Read the model definition and answer for the solid it produces. Units are mm, in the model's axes. A direction names the side the tool comes from. Give positions to 0.01 mm unless a question says otherwise; leave off trailing zeros. Order: outer loops, then holes, each group sorted by start corner. A loop starts at its lowest first (then second) coordinate and runs counter-clockwise, first axis right, second up.
Item 1: Find the intervals of material crossed by line 1 along Z through (x, y) = (-67, 215); line 2 along Z through (x, y) = (-125, 37); line 3 along Y through (x, z) = (-145.5, -16.5), in increasing order.
Item 2: Given pin 1 Ø2 at (x, y) = (-131, 12) entering from -Z; pin 2 Ø15.5 at (x, z) = (-147, -16) entering from +Y; pin 3 Ø1 at (y, z) = (132.5, -10.5) entering from +X; pin 4 Ø1.5 at (x, y) = (-107, 18) entering from +Z, each flat-ended and moving along its own axis, determine where each tip first touches the part or whether it passes through.
Item 3: A cutting plane is placed at C-C (y = 175). Write down the section's boundary in (x, z), plus the area to 3 significant figures.
Item 4: A cutting plane is placed at A-A (x = -61). Write down the section's boundary in (y, z), plus the area to 3 significant figures.
Item 5: A cutting plane is placed at B-B (z = -15.5). Write down the section's boundary in (x, y).
Item 6: Which of the six approach directions +Z, -Z, +X, -X, +Y, -Y give full straight-line access (tool end or side, diameter ignored) to faces 1 (the face through (-146, 108.104, -11)), 2 (the face through (-146, 106.89, -12)), 3 (the face through (-30.09, 196, -12))?
Item 7: A cutting plane is placed at D-D (z = 15). Write down the section's boundary in (x, y).
from build123d import *

# Parameters (mm, degrees)
BASE_FLANGE1_DEPTH            = 1.21412
SKETCH19_W                    = 150.565156201
SKETCH19_H                    = 181.162980563
CUT_EXTRUDE2_DEPTH            = 5
EDGE_FLANGE5_START            = 106.282964216
EDGE_FLANGE5_DEPTH            = 181.770040563
EDGE_FLANGE5_2_DEPTH          = 0.60706
EDGE_FLANGE5_START_2          = 106.890024216
EDGE_FLANGE5_3_DEPTH          = 181.162980563
EDGE_FLANGE6_STRIP_W          = 7.39648
EDGE_FLANGE6_STRIP_H          = 1.21412
EDGE_FLANGE6_STRIP_CUT_DEPTH  = 181.162980563
EDGE_FLANGE6_DEPTH            = 181.162980563
EDGE_FLANGE7_STRIP_W          = 7.39648
EDGE_FLANGE7_STRIP_H          = 1.21412
EDGE_FLANGE7_STRIP_CUT_DEPTH  = 14.216886025
EDGE_FLANGE7_RELIEF_W         = 8.00354
EDGE_FLANGE7_RELIEF_H         = 0.60706
EDGE_FLANGE7_RELIEF_CUT_DEPTH = 1.21412
EDGE_FLANGE7_DEPTH            = 14.216886025
SKETCH29_R                    = 2.5
CUT_EXTRUDE3_DEPTH            = 5
EDGE_FLANGE8_START            = -92.476413081
EDGE_FLANGE8_DEPTH            = 53.21412
EDGE_FLANGE8_2_DEPTH          = 0.60706
EDGE_FLANGE8_START_2          = -39.869353081
EDGE_FLANGE8_3_DEPTH          = 0.60706
EDGE_FLANGE8_START_3          = -91.869353081
EDGE_FLANGE8_4_DEPTH          = 52
EDGE_FLANGE8_START_4          = 58
EDGE_FLANGE8_5_DEPTH          = 2.895111402
SKETCH34_R                    = 2.25
CUT_EXTRUDE6_DEPTH            = 10


with BuildPart() as part:
    # Base-Flange1: sheet metal written as solids
    # Sketch1 → Base-Flange1 (new body)
    with BuildSketch(Plane.XY):
        with BuildLine():
            Line((-96.869353081, -33.474110531), (-176.869353081, -33.474110531))
            ThreePointArc((-176.869353081, -33.474110531), (-180.404886987, -32.009644437), (-181.869353081, -28.474110531))
            Line((-181.869353081, -28.474110531), (-181.869353081, 288.053004779))
            Line((-181.869353081, 288.053004779), (-18.770502539, 288.053004779))
            Line((-18.770502539, 288.053004779), (-18.770502539, 81.588857582))
            ThreePointArc((-18.770502539, 81.588857582), (-21.699434728, 74.51778977), (-28.770502539, 71.588857582))
            Line((-28.770502539, 71.588857582), (-91.869353081, 71.588857582))
            Line((-91.869353081, 71.588857582), (-91.869353081, -28.474110531))
            ThreePointArc((-91.869353081, -28.474110531), (-93.333819175, -32.009644437), (-96.869353081, -33.474110531))
        make_face()
    extrude(amount=-BASE_FLANGE1_DEPTH)

    # Sketch19 → Cut-Extrude2 (cut)
    with BuildSketch(Plane(origin=(0, 0, -1.21412), x_dir=(-1, 0, 0), z_dir=(0, 0, -1))):
        with Locations((106.586774981, 197.471514497)):
            Rectangle(SKETCH19_W, SKETCH19_H)
    extrude(amount=-CUT_EXTRUDE2_DEPTH, mode=Mode.SUBTRACT)

    # Edge-Flange5: read off the stored shape, not the designer's step
    # Edge-Flange5 outline → Edge-Flange5 (cut)
    with BuildSketch(Plane(origin=(0, 0, 0), x_dir=(1, 0, 0), z_dir=(0, 1, 0)).offset(EDGE_FLANGE5_START)):
        with BuildLine():
            Line((-31.30419688, 0), (-28.82007688, 0))
            ThreePointArc((-28.82007688, 0), (-30.04808742, 0.324758454), (-30.955012985, 1.21412))
            Line((-30.955012985, 1.21412), (-31.30419688, 1.21412))
            Line((-31.30419688, 1.21412), (-31.30419688, 0))
        make_face()
    extrude(amount=EDGE_FLANGE5_DEPTH, mode=Mode.SUBTRACT)

    # Edge-Flange5 2 outline → Edge-Flange5 2 (cut)
    with BuildSketch(Plane(origin=(0, 0, 0), x_dir=(1, 0, 0), z_dir=(0, 1, 0)).offset(EDGE_FLANGE5_START)):
        with BuildLine():
            Line((-28.21301688, 0), (-28.21301688, 1.21412))
            Line((-28.21301688, 1.21412), (-30.955012985, 1.21412))
            ThreePointArc((-30.955012985, 1.21412), (-30.04808742, 0.324758454), (-28.82007688, 0))
            Line((-28.82007688, 0), (-28.21301688, 0))
        make_face()
    extrude(amount=EDGE_FLANGE5_2_DEPTH, mode=Mode.SUBTRACT)

    # Edge-Flange5 3 outline → Edge-Flange5 3 (add)
    with BuildSketch(Plane(origin=(0, 0, 0), x_dir=(1, 0, 0), z_dir=(0, 1, 0)).offset(EDGE_FLANGE5_START_2)):
        with BuildLine():
            Line((-30.955012985, 1.21412), (-28.82007688, 1.21412))
            ThreePointArc((-28.82007688, 1.21412), (-29.718102492, 1.586094388), (-30.09007688, 2.48412))
            Line((-30.09007688, 2.48412), (-30.09007688, 24))
            Line((-30.09007688, 24), (-31.30419688, 24))
            Line((-31.30419688, 24), (-31.30419688, 2.48412))
            ThreePointArc((-31.30419688, 2.48412), (-31.215310653, 1.825555388), (-30.955012985, 1.21412))
        make_face()
    extrude(amount=EDGE_FLANGE5_3_DEPTH)

    # Edge-Flange6: sheet metal written as solids
    # Edge-Flange6 strip (on a plane across the edge) → Edge-Flange6 strip cut (cut)
    with BuildSketch(Plane(origin=(-31.30419688, 288.053004779, -24), x_dir=(0, 0, 1), z_dir=(0, -1, 0))):
        with Locations((-1.21412, -0.60706)):
            Rectangle(EDGE_FLANGE6_STRIP_W, EDGE_FLANGE6_STRIP_H)
    extrude(amount=EDGE_FLANGE6_STRIP_CUT_DEPTH, mode=Mode.SUBTRACT)

    # Edge-Flange6 section (on a plane across the edge) → Edge-Flange6 (add)
    with BuildSketch(Plane(origin=(-31.30419688, 288.053004779, -24), x_dir=(0, 0, 1), z_dir=(0, -1, 0))):
        with BuildLine():
            Line((0, 1.27), (0, 121.48412))
            Line((0, 121.48412), (1.21412, 121.48412))
            Line((1.21412, 121.48412), (1.21412, 1.27))
            ThreePointArc((1.21412, 1.27), (1.586094388, 0.371974388), (2.48412, 0))
            Line((2.48412, 0), (2.48412, -1.21412))
            ThreePointArc((2.48412, -1.21412), (0.727581903, -0.486538097), (0, 1.27))
        make_face()
    extrude(amount=EDGE_FLANGE6_DEPTH)

    # Edge-Flange7: sheet metal written as solids
    # Edge-Flange7 strip (on a plane across the edge) → Edge-Flange7 strip cut (cut)
    with BuildSketch(Plane(origin=(-152.78831688, 106.890024216, -22.78588), x_dir=(0, 1, 0), z_dir=(1, 0, 0))):
        with Locations((-1.21412, -0.60706)):
            Rectangle(EDGE_FLANGE7_STRIP_W, EDGE_FLANGE7_STRIP_H)
    extrude(amount=EDGE_FLANGE7_STRIP_CUT_DEPTH, mode=Mode.SUBTRACT)

    # Edge-Flange7 relief (on the sheet) → Edge-Flange7 relief cut (cut)
    with BuildSketch(Plane(origin=(-152.78831688, 109.374144216, -22.78588), x_dir=(0, 1, 0), z_dir=(0, 0, 1))):
        with Locations((-3.39471, -14.520416025)):
            Rectangle(EDGE_FLANGE7_RELIEF_W, EDGE_FLANGE7_RELIEF_H)
    extrude(amount=-EDGE_FLANGE7_RELIEF_CUT_DEPTH, mode=Mode.SUBTRACT)

    # Edge-Flange7 section (on a plane across the edge) → Edge-Flange7 (add)
    with BuildSketch(Plane(origin=(-152.78831688, 106.890024216, -22.78588), x_dir=(0, 1, 0), z_dir=(1, 0, 0))):
        with BuildLine():
            Line((0, 1.27), (0, 21.28588))
            Line((0, 21.28588), (1.21412, 21.28588))
            Line((1.21412, 21.28588), (1.21412, 1.27))
            ThreePointArc((1.21412, 1.27), (1.586094388, 0.371974388), (2.48412, 0))
            Line((2.48412, 0), (2.48412, -1.21412))
            ThreePointArc((2.48412, -1.21412), (0.727581903, -0.486538097), (0, 1.27))
        make_face()
    extrude(amount=EDGE_FLANGE7_DEPTH)

    # Sketch29 → Cut-Extrude3 (cut)
    with BuildSketch(Plane.XY):
        with Locations((-157.869353081, 45.8541873)):
            Circle(SKETCH29_R)
        with Locations((-115.869353081, 45.8541873)):
            Circle(SKETCH29_R)
        with Locations((-157.869353081, -6.1458127)):
            Circle(SKETCH29_R)
        with Locations((-115.869353081, -6.1458127)):
            Circle(SKETCH29_R)
        with BuildLine():
            Line((-120.869353081, -18.100802087), (-141.694922457, -18.100802087))
            ThreePointArc((-141.694922457, -18.100802087), (-147.149911844, -12.6458127), (-141.694922457, -7.190823313))
            Line((-141.694922457, -7.190823313), (-120.869353081, -7.190823313))
            ThreePointArc((-120.869353081, -7.190823313), (-115.414363694, -12.6458127), (-120.869353081, -18.100802087))
        make_face()
    extrude(amount=-CUT_EXTRUDE3_DEPTH, mode=Mode.SUBTRACT)

    # Edge-Flange8: read off the stored shape, not the designer's step
    # Edge-Flange8 outline → Edge-Flange8 (cut)
    with BuildSketch(Plane.YZ.offset(EDGE_FLANGE8_START)):
        with BuildLine():
            Line((71.588857582, -1.21412), (73.732144579, -1.21412))
            ThreePointArc((73.732144579, -1.21412), (72.585105614, -0.933441351), (71.697272603, -0.154832697))
            Line((71.697272603, -0.154832697), (71.588857582, 0))
            Line((71.588857582, 0), (71.588857582, -1.21412))
        make_face()
    extrude(amount=EDGE_FLANGE8_DEPTH, mode=Mode.SUBTRACT)

    # Edge-Flange8 2 outline → Edge-Flange8 2 (cut)
    with BuildSketch(Plane.YZ.offset(EDGE_FLANGE8_START)):
        with BuildLine():
            Line((74.339204579, -1.21412), (74.339204579, 0))
            Line((74.339204579, 0), (71.588857582, 0))
            Line((71.588857582, 0), (71.697272603, -0.154832697))
            ThreePointArc((71.697272603, -0.154832697), (72.585105614, -0.933441351), (73.732144579, -1.21412))
            Line((73.732144579, -1.21412), (74.339204579, -1.21412))
        make_face()
    extrude(amount=EDGE_FLANGE8_2_DEPTH, mode=Mode.SUBTRACT)

    # Edge-Flange8 3 outline → Edge-Flange8 3 (cut)
    with BuildSketch(Plane.YZ.offset(EDGE_FLANGE8_START_2)):
        with BuildLine():
            Line((74.339204579, -1.21412), (74.339204579, 0))
            Line((74.339204579, 0), (71.588857582, 0))
            Line((71.588857582, 0), (71.697272603, -0.154832697))
            ThreePointArc((71.697272603, -0.154832697), (72.585105614, -0.933441351), (73.732144579, -1.21412))
            Line((73.732144579, -1.21412), (74.339204579, -1.21412))
        make_face()
    extrude(amount=EDGE_FLANGE8_3_DEPTH, mode=Mode.SUBTRACT)

    # Edge-Flange8 4 outline → Edge-Flange8 4 (add)
    with BuildSketch(Plane.YZ.offset(EDGE_FLANGE8_START_3)):
        with BuildLine():
            Line((71.588857582, 0), (73.732144579, 0))
            ThreePointArc((73.732144579, 0), (73.14572384, 0.143496242), (72.691821483, 0.541557926))
            Line((72.691821483, 0.541557926), (47.529257546, 36.477423457))
            Line((47.529257546, 36.477423457), (46.534708666, 35.781032834))
            Line((46.534708666, 35.781032834), (71.588857582, 0))
        make_face()
    extrude(amount=EDGE_FLANGE8_4_DEPTH)

    # Edge-Flange8 5 outline → Edge-Flange8 5 (cut)
    with BuildSketch(Plane(origin=(0, 0, 0), x_dir=(1, 0, 0), z_dir=(0, 0.8191520442889886, 0.5735764363510508)).offset(EDGE_FLANGE8_START_4)):
        with BuildLine():
            ThreePointArc((-39.869353081, 2.381106171), (-41.333819175, -1.154427735), (-44.869353081, -2.618893829))
            Line((-44.869353081, -2.618893829), (-39.869353081, -2.61889383))
            Line((-39.869353081, -2.61889383), (-39.869353081, 2.381106171))
        make_face()
        with BuildLine():
            Line((-91.869353081, -2.61889383), (-86.869353081, -2.618893829))
            ThreePointArc((-86.869353081, -2.618893829), (-90.404886987, -1.154427735), (-91.869353081, 2.381106171))
            Line((-91.869353081, 2.381106171), (-91.869353081, -2.61889383))
        make_face()
    extrude(amount=EDGE_FLANGE8_5_DEPTH, mode=Mode.SUBTRACT)

    # Sketch34 → Cut-Extrude6 (cut)
    with BuildSketch(Plane(origin=(0, 49.031393336, 34.332151223), x_dir=(1, 0, 0), z_dir=(0, 0.8191520442889887, 0.5735764363510506))):
        with Locations(Location((-80.981806948, 37.381106171, 0), (0, 0, 270))):
            Circle(SKETCH34_R)
        with Locations(Location((-49.861806948, 37.381106171, 0), (0, 0, 270))):
            Circle(SKETCH34_R)
    extrude(amount=-CUT_EXTRUDE6_DEPTH, mode=Mode.SUBTRACT)


solid = part.part
Response values:
1. line 1: z = -24 to -22.79
1. line 2: z = -1.21 to 0
1. line 3: y = 106.89 to 108.1
2. pin 1: stops at z = -1.21
2. pin 2: stops at y = 288.05
2. pin 3: stops at x = -30.09
2. pin 4: stops at z = 0
3. outline: (-152.79, -24) - (-32.57, -24) arc R2.48 ccw to (-30.09, -21.52) - (-30.09, -2.48) arc R1.27 cw to (-28.82, -1.21) - (-18.77, -1.21) - (-18.77, 0) - (-28.82, 0) arc R2.48 ccw to (-31.3, -2.48) - (-31.3, -21.52) arc R1.27 cw to (-32.57, -22.79) - (-152.79, -22.79) - close
3. area: 188 mm2
4. outline: (46.53, 35.78) - (71.7, -0.15) arc R2.48 ccw to (73.73, -1.21) - (106.89, -1.21) - (106.89, 0) - (73.73, 0) arc R1.27 cw to (72.69, 0.54) - (47.53, 36.48) - close; (106.89, -24) - (288.05, -24) - (288.05, -22.79) - (106.89, -22.79) - close
4. area: 316 mm2
5. outline: (-152.79, 106.89) - (-138.57, 106.89) - (-138.57, 108.1) - (-152.79, 108.1) - close; (-31.3, 106.89) - (-30.09, 106.89) - (-30.09, 288.05) - (-31.3, 288.05) - close
6. face 1: +Z, -X, +Y
6. face 2: -Z, +X, -X, -Y
6. face 3: -Z, +X, +Y, -Y
7. outline: (-91.87, 61.09) - (-39.87, 61.09) - (-39.87, 62.57) - (-91.87, 62.57) - close
